Input: dimensioned drawing with shaded views. Units: mm. Origin: part minimum x, y, z. A direction names the side the tool comes from. Round coordinates to 2 decimals unless told otherwise and drop trailing zeros. Loops run counter-clockwise (first coordinate to the right, second up) from the corner with the lowest first, then second, coordinate; pieces in that order, holes last.
Item 1: Section query B-B on x = 55. Return loops of the section in (y, z).
Item 2: Section query C-C on y = 26. Return loops of the section in (x, z).
Item 3: First-contact query: P1, Ø10, axis at y = 23, z = 27.5, coming from the +X side; P2, Ø3, axis at y = 17.5, z = 45, coming from the +X side; P3, Ø21.5, axis at x = 55, z = 25, coming from the -Y side; P4, Ø1, axis at x = 51.5, z = 7, coming from the +Y side. Flat tips, straight axial feed; report the tip coordinate or a pass-through.
Item 4: Ray query, L1, parallel to X at y = 2.25, z = 25; L2, parallel to Z at x = 33, y = 30.5; L3, parallel to Y at x = 69, z = 37.5. Return the intervals inside material, ascending.
Item 5: Section query A-A on z = 25. Return loops of the section in (x, y).
Item 6: Section query D-D on x = 23. Return loops of the section in (y, z), then the cut area to 3 significant figures.
Item 7: Pull-direction query (Z, two-part tool) for the marked faces 4, 5, 6 and 7; classes: released by +Z, released by -Z, zero draft, split by the parting line, or undercut.
Item 8: Access query for the marked faces 1, 2 and 3. Directions: +Z, -Z, +X, -X, +Y, -Y. A direction counts if a zero-diameter tool reaches every point of the face in a straight line with its end or side. Return the directions, or none.
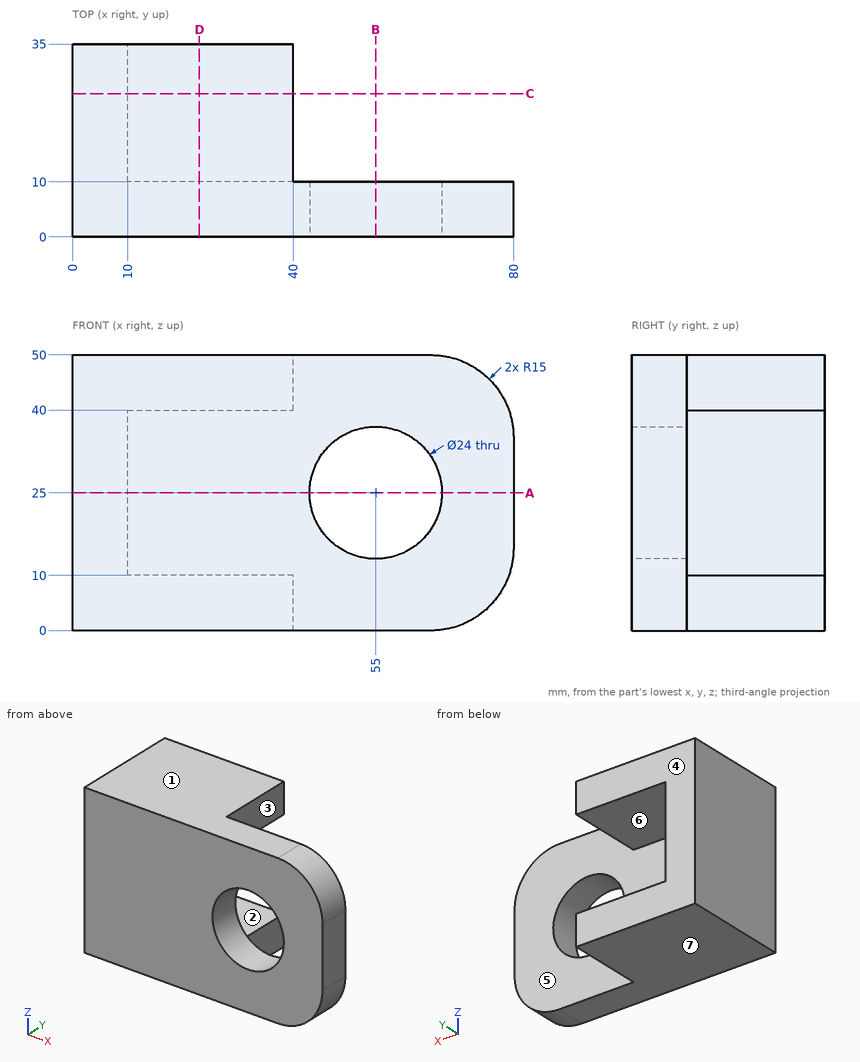
Data:
1. outline: (0, 0) - (10, 0) - (10, 13) - (0, 13) - close; (0, 37) - (10, 37) - (10, 50) - (0, 50) - close
2. outline: (0, 0) - (40, 0) - (40, 10) - (10, 10) - (10, 40) - (40, 40) - (40, 50) - (0, 50) - close
3. P1: stops at x = 10
3. P2: stops at x = 40
3. P3: passes through
3. P4: stops at y = 10
4. L1: x = 0 to 43, 67 to 80
4. L2: z = 0 to 10, 40 to 50
4. L3: y = 0 to 10
5. outline: (0, 0) - (43, 0) - (43, 10) - (10, 10) - (10, 35) - (0, 35) - close; (67, 0) - (80, 0) - (80, 10) - (67, 10) - close
6. outline: (0, 0) - (35, 0) - (35, 10) - (10, 10) - (10, 40) - (35, 40) - (35, 50) - (0, 50) - close
6. area: 1,000 mm2
7. face 4: zero draft
7. face 5: undercut
7. face 6: undercut
7. face 7: released by -Z
8. face 1: +Z, +X, -X, +Y, -Y
8. face 2: +X, +Y
8. face 3: +Z, -Z, +X, +Y
